Autodesk Fusion 360 part; units mm, degrees
sketch "Sketch1" plane through (0, 0, 0) normal (0, 0, 1) x (1, 0, 0)
  line L0 (0, 0) -> (25, 0)
  line L1 (25, 0) -> (25, 25)
  line L2 (25, 25) -> (0, 25)
  line L3 (0, 25) -> (0, 5)
  line L4 (0, 0) -> (-20, 0)
  line L5 (-20, 0) -> (-20, 5)
  line L6 (-20, 5) -> (0, 5)
extrude "Extrude1" add sketch "Sketch1" along normal blind 1
sketch "Sketch2" plane through (0, 0, 1) normal (0, 0, 1) x (-1, 0, 0)
  line L0 (20, 0) -> (-25, 0)
  line L1 (-25, 0) -> (-25, -25)
  line L2 (-25, -25) -> (0, -25)
  line L3 (0, -25) -> (0, -5)
  line L4 (0, -5) -> (20, -5)
  line L5 (20, -5) -> (20, 0)
  line L6 (-1, -1) -> (-24, -1)
  line L7 (-24, -1) -> (-24, -24)
  line L8 (-24, -24) -> (-1, -24)
  line L9 (-1, -24) -> (-1, -1)
  line L10 (0, -5) -> (0, 0)
extrude "Extrude2" add sketch "Sketch2" along normal blind 4
sketch "Sketch3" plane through (0, 0, 5) normal (0, 0, 1) x (-1, 0, 0)
  line L0 (-1, -1) -> (-1, -24)
  line L1 (-1, -24) -> (-24, -24)
  line L2 (-24, -24) -> (-24, -1)
  line L3 (-24, -1) -> (-1, -1)
  line L4 (20, -5) -> (20, 0)
  line L5 (20, 0) -> (-25, 0)
  line L6 (-25, 0) -> (-25, -25)
  line L7 (-25, -25) -> (0, -25)
  line L8 (0, -25) -> (0, -5)
  line L9 (0, -5) -> (20, -5)
  line L10 (0, -5) -> (0, 0)
extrude "Extrude3" add sketch "Sketch3" along normal blind 10 contours L5 L6 L7 L8 L10
sketch "Sketch4" plane through (-20, 0, 0) normal (-1, 0, 0) x (0, -1, 0)
  line L0 (-5, 0) -> (0, 0)
  line L1 (0, 0) -> (0, 5)
  line L2 (0, 5) -> (-5, 5)
  line L3 (-5, 5) -> (-5, 0)
  line L4 (-4, 4) -> (-1, 4)
  line L5 (-1, 4) -> (-1, 1)
  line L6 (-1, 1) -> (-4, 1)
  line L7 (-4, 1) -> (-4, 4)
extrude "Extrude4" cut sketch "Sketch4" against normal blind 23 contours L4 L5 L6 L7
sketch "Sketch5" plane through (0, 1, 0) normal (0, 1, 0) x (-1, 0, 0)
  line L0 (-24, 1) -> (20, 1)
  line L1 (20, 1) -> (20, 4)
  line L2 (20, 4) -> (-1, 4)
  line L3 (-1, 4) -> (-1, 15)
  line L4 (-1, 15) -> (-24, 15)
  line L5 (-24, 15) -> (-24, 1)
  line L6 (-1, 4) -> (-24, 4)
  line L7 (-24, 4) -> (-24, 5)
  line L8 (-24, 5) -> (-1, 5)
  line L9 (-1, 4) -> (-1, 5)
extrude "Extrude5" add sketch "Sketch5" along normal blind 23 contours L3 L5 L6 L7 L8 L9
sketch "Sketch6" plane through (0, 5, 0) normal (0, 1, 0) x (-1, 0, 0)
  line L0 (0, 0) -> (20, 0)
  line L1 (20, 0) -> (20, 5)
  line L2 (20, 5) -> (0, 5)
  line L3 (0, 5) -> (0, 0)
  line L4 (0, 4) -> (1.5, 4)
  line L5 (1.5, 4) -> (1.5, 2.5)
  line L6 (1.5, 2.5) -> (0, 2.5)
  line L7 (0, 4) -> (0, 2.5)
extrude "Extrude6" cut sketch "Sketch6" against normal blind 2 contours L3 L4 L5 L6 L7
sketch "Sketch7" plane through (-20, 0, 0) normal (-1, 0, 0) x (0, -1, 0)
  line L0 (-1, 4) -> (-1, 1)
  line L1 (-1, 1) -> (-4, 1)
  line L2 (-4, 1) -> (-4, 4)
  line L3 (-4, 4) -> (-1, 4)
  line L4 (-5, 0) -> (0, 0)
  line L5 (0, 0) -> (0, 5)
  line L6 (0, 5) -> (-5, 5)
  line L7 (-5, 5) -> (-5, 0)
  line L8 (-5, 1) -> (0, 1)
extrude "Extrude7" add sketch "Sketch7" along normal blind 6 contours L1 L4 L5 L7 L8
sketch "Sketch8" plane through (0, 0, 1) normal (0, 0, 1) x (-1, 0, 0)
  line L0 (20, -1) -> (-24, -1)
  line L1 (-24, -1) -> (-24, -24)
  line L2 (-24, -24) -> (-1, -24)
  line L3 (-1, -24) -> (-1, -4)
  line L4 (-1, -4) -> (20, -4)
  line L5 (20, -4) -> (20, -5)
  line L6 (20, -5) -> (26, -5)
  line L7 (26, -5) -> (26, 0)
  line L8 (26, 0) -> (20, 0)
  line L9 (20, 0) -> (20, -1)
  line L10 (20, -1) -> (24, -1)
  line L11 (24, -1) -> (24, -4)
  line L12 (24, -4) -> (20, -4)
extrude "Extrude8" add sketch "Sketch8" along normal blind 4 contours L5 L6 L7 L8 L9 L10 L11 L12
extrude "Extrude9" cut 1 faces at (-26, 3.3333, 1.6667) along direction (1, 0, 0) blind 1
extrude "Extrude10" add 1 faces at (-20, 2, 4.3333) along direction (-1, 0, 0) blind 1
sketch "Sketch9" plane through (0, 0, 5) normal (0, 0, 1) x (-1, 0, 0)
  line L0 (21, -1) -> (24, -1)
  line L1 (24, -1) -> (24, -4)
  line L2 (24, -4) -> (21, -4)
  line L3 (21, -4) -> (21, -1)
  line L4 (25, -5) -> (25, 0)
  line L5 (25, 0) -> (0, 0)
  line L6 (0, 0) -> (0, -5)
  line L7 (0, -5) -> (25, -5)
  line L8 (20, 0) -> (20, -5)
extrude "Extrude11" add sketch "Sketch9" along normal blind 15 contours L4 L5 L7 L8
extrude "Extrude12" cut 1 faces at (16.3333, 0.3333, 15) along direction (0, 0, -1) blind 6
Input: part model. Units: mm. Frame: model coordinates. A direction names the side the tool comes from. Round coordinates to 2 decimals unless told otherwise and drop trailing zeros. Write each loop counter-clockwise with the first axis right and the second up, starting at its lowest first coordinate (ties: lowest second). Pieces come first, ordered by that corner, then holes. Notation, with made-up numbers: (71.5, 65) - (92.5, 65) arc R22 ccw to (92.5, 97) - close; hole circle Ø2 at (13, 44.5). An arc over 180 degrees is marked (long way). Write item = value, one per line.
(1) Pull-direction query (X, two-part tool) for faces 1 (the flat face through (0, 0, 3)), 2 (the flat face through (25, 12, 4)), 3 (the flat face through (-0.8, 4.5, 2.5)); classes: +X half, -X half, draft (parallel to the pull), parting line (faces both ways), or undercut.
Geometry check:
face_1 = draft
face_2 = +X half
face_3 = undercut
(2) Section query B-B on z = 7.25. Output: boundary loops of the cut face in (x, y).
Geometry check:
outline = (-25, 0) - (-20, 0) - (-20, 5) - (-25, 5) - close; (0, 0) - (25, 0) - (25, 25) - (0, 25) - close; hole (-24, 1) - (-21, 1) - (-21, 4) - (-24, 4) - close; hole (1, 1) - (24, 1) - (24, 24) - (1, 24) - close
(3) Section query A-A on y = 6.75. Output: boundary loops of the cut face in (x, z).
Geometry check:
outline = (0, 0) - (25, 0) - (25, 9) - (24, 9) - (24, 5) - (1, 5) - (1, 9) - (0, 9) - close; hole (1, 1) - (24, 1) - (24, 4) - (1, 4) - close
(4) Contact query for flat-ended pins moving along their axis: pin 1 Ø2.5 at (x, y) = (-11.5, 2) entering from +Z; pin 2 Ø2.5 at (y, z) = (13, 5.5) entering from -X; pin 3 Ø12.5 at (x, y) = (11.5, 6.5) entering from +Z; pin 4 Ø6 at (y, z) = (13, 14) entering from -X. Output: stop coordinate, or through.
Geometry check:
pin_1 = 5
pin_2 = 0
pin_3 = 9
pin_4 = through
(5) Section query D-D on z = 14. Output: boundary loops of the cut face in (x, y).
Geometry check:
outline = (-25, 0) - (-20, 0) - (-20, 5) - (-25, 5) - close; hole (-24, 1) - (-21, 1) - (-21, 4) - (-24, 4) - close
(6) Section query C-C on x = -12. Output: boundary loops of the cut face in (y, z), then the cut area to 3 significant figures.
Geometry check:
outline = (0, 0) - (5, 0) - (5, 5) - (0, 5) - close; hole (1, 1) - (4, 1) - (4, 4) - (1, 4) - close
area = 16.0 mm^2
(7) Material intervals for probe 1 along Z at (x, y) = (-6, 1.25); probe 2 along Y at (x, z) = (4.5, 6.25); probe 3 along Z at (x, y) = (0.5, 1.75), sorted ascending.
Geometry check:
probe_1 = 0 to 1, 4 to 5
probe_2 = 0 to 1, 24 to 25
probe_3 = 0 to 1, 4 to 9
(8) Access query for faces 4 (the flat face through (12, 13, 4)), 5 (the flat face through (6, 10, 0)), 6 (the flat face through (13, 12, 5)), 7 (the flat face through (-18, 5, 3)). Directions: +Z, -Z, +X, -X, +Y, -Y. A direction counts if a zero-diameter tool reaches every point of the face in a straight line with its end or side. Return the directions, or none.
Geometry check:
face_4 = none
face_5 = -Z, +X, -X, +Y, -Y
face_6 = +Z
face_7 = +Z, -Z, -X, +Y
